Geometry check sheet. Reference: the model listing, model coordinates, mm. Face numbers are marked on the shaded views. Give positions to 0.01 mm unless a question says otherwise; leave off trailing zeros. Order: outer loops, then holes, each group sorted by start corner. A loop starts at its lowest first (then second) coordinate and runs counter-clockwise, first axis right, second up. Notation, with made-up numbers: M 1,77.5 L 23,77.5 A10 cw 23,93.5 Z; hole C 34.25,29.5 d9. An arc over 180 degrees is marked long. Answer as a JSON object with one key per item and string values. Group by question number.
Autodesk Inventor part; units mm, degrees
ref_plane "YZ Plane" through (0, 0, 0) normal (1, 0, 0) x (0, 1, 0)
ref_plane "XZ Plane" through (0, 0, 0) normal (0, 1, 0) x (-1, 0, 0)
ref_plane "XY Plane" through (0, 0, 0) normal (0, 0, 1) x (1, 0, 0)
sketch "Sketch1" plane through (0, 0, 0) normal (0, 0, 1) x (1, 0, 0)
  line L0 (2.35, 1.3568) -> (2.35, -1.3568)
  line L1 (2.35, -1.3568) -> (0, -2.7135)
  line L2 (0, -2.7135) -> (-2.35, -1.3568)
  line L3 (-2.35, 1.3568) -> (-2.35, -1.3568)
  line L4 (-2.35, 1.3568) -> (0, 2.7135)
  line L5 (0, 2.7135) -> (2.35, 1.3568)
  circle A0 centre (0, 0) radius 2.7135 construction
  line L6 (0, 29.0365) -> (0, -7.2493) construction
  line L7 (0, -14.5064) -> (0, 36.2936)
  line L8 (-3.799, 0) -> (3.799, 0)
  dimension "d0" = 5.4271
  dimension "d20" = 4.7
  dimension "d21" = 2.7136
extrude "Hexagon1" add sketch "Sketch1" along normal blind 5
hole "Hole1" at (0, 0, 0) direction (0, 0, 1) diameter 2.459 end through all
properties part number "Spacer-M3-FF-05" material "Brass, Soft Yellow, Welded"
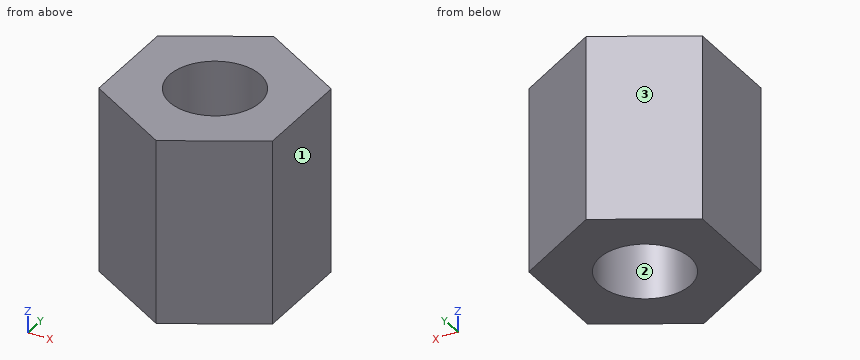
1. Release check for a two-part mould opening along X. For the marked faces 1, 2 and 3 record: released by +X, released by -X, zero draft, split by the parting line, or undercut.
2. Cross-section at C-C (x = 0.55). Record the cut outline in (y, z).
3. Cross-section at D-D (y = 2.3). Record the cut outline in (x, z).
4. Thickness scan on line 1 along X through (y, z) = (0, 1.55); line 2 along X through (y, z) = (-0.55, 1.2); line 3 along Y through (x, z) = (1.05, 1.5). Record the ranges inside material, lowest first. Write a range as [from, to].
5. Cross-section at A-A (y = 0). Record the cut outline in (x, z).
6. Cross-section at B-B (z = 4.15). Record the cut outline in (x, y), and give its area (3 significant figures).
Report:
{
 "1": {"face 1": "released by +X", "face 2": "undercut", "face 3": "released by -X"},
 "2": {"outline": "M -2.4,0 L -1.1,0 L -1.1,5 L -2.4,5 Z; M 1.1,0 L 2.4,0 L 2.4,5 L 1.1,5 Z"},
 "3": {"outline": "M -0.72,0 L 0.72,0 L 0.72,5 L -0.72,5 Z"},
 "4": {"line 1": "x = [-2.35, -1.23], [1.23, 2.35]", "line 2": "x = [-2.35, -1.1], [1.1, 2.35]", "line 3": "y = [-2.11, -0.64], [0.64, 2.11]"},
 "5": {"outline": "M -2.35,0 L -1.23,0 L -1.23,5 L -2.35,5 Z; M 1.23,0 L 2.35,0 L 2.35,5 L 1.23,5 Z"},
 "6": {"outline": "M -2.35,-1.36 L 0,-2.71 L 2.35,-1.36 L 2.35,1.36 L 0,2.71 L -2.35,1.36 Z; hole C 0,0 d2.46", "area": "14.4 mm2"}
}
